```python
from build123d import *

# Parameters (mm, degrees)
SKETCH2_R = 65


with BuildPart() as part:
    # Sweep1: sweep along a path in Sketch1
    with BuildLine(Plane(origin=(0, 0, 0), x_dir=(0, 0, -1), z_dir=(1, 0, 0))) as sweep1_path:
        Line((-50, 0), (50, 0))
        Line((50, 0), (50, 120))
    # Sketch2 → Sweep1 (sweep)
    with BuildSketch(Plane.XY.offset(50)):
        Circle(SKETCH2_R)
    sweep1 = sweep(path=sweep1_path.line, transition=Transition.RIGHT)

    # Mirror1: Sweep1 across plane
    add(sweep1.mirror(Plane.XY.offset(-50)))


solid = part.part
```
Can you work these out from the model? Positions are in its coordinate system, mm. A direction names the side the tool comes from. Coordinates: 2 decimals unless noted, no trailing zeros. Loops run counter-clockwise (first coordinate to the right, second up) from the corner with the lowest first, then second, coordinate; pieces in that order, holes last. Notation, with made-up numbers: (81, 28) -> (105, 28) arc R21 cw to (105, 35) -> close; hole circle Ø3 at (-28, 41.5). An arc over 180 degrees is marked (long way). Answer as a JSON object with one key per item and string values.
1) Imagine slicing it at D-D (y = 68). Please give me the cut outline in (x, z).
Results:
{"outline": "circle Ø130 at (0, -50)"}
2) Imagine slicing it at B-B (x = 0). Please give me the cut outline in (y, z), then the cut area to 4 significant figures.
Results:
{"outline": "(-65, -150) -> (65, -150) -> (65, -115) -> (120, -115) -> (120, 15) -> (65, 15) -> (65, 50) -> (-65, 50) -> close", "area": "33,150 mm^2"}
3) Imagine slicing it at C-C (z = 6). Please give me the cut outline in (x, y).
Results:
{"outline": "(-33, 56) arc R65 ccw (long way) to (33, 56) -> (33, 120) -> (-33, 120) -> close"}
4) For faces 1 (the face through (1, 120, -49)), 2 (the face through (-47.91, 74.17, -93.93)), which set-ups out of +Z, -Z, +X, -X, +Y, -Y let a thin tool reach every point of the face, with its end or its side?
Results:
{"face 1": "+Z, -Z, +X, -X, +Y", "face 2": "+Y"}
5) If I drill on line 1 (X direction, y = 76.5, z = -50.5); line 2 (Y direction, x = 30, z = -64); line 3 (Y direction, x = -51.5, z = 3.5), over which ranges is the centre line in solid material (lowest first)?
Results:
{"line 1": "x = -65 to 65", "line 2": "y = -57.66 to 120", "line 3": "y = -39.66 to 39.66"}
6) Imagine slicing it at A-A (y = 44). Please give me the cut outline in (x, z).
Results:
{"outline": "(-47.84, -150) -> (47.84, -150) -> (47.84, -94) arc R65 ccw to (47.84, -6) -> (47.84, 50) -> (-47.84, 50) -> (-47.84, -6) arc R65 ccw to (-47.84, -94) -> close"}
7) For P1, Ø5, axis at x = 7.5, z = -5, coming from the -Y side; P2, Ø10, axis at x = 45.5, z = 2, coming from the -Y side; P3, Ø10, axis at y = -33, z = -120.5, coming from the -X side, each with a flat end and sliding along its axis, tell me the tip position at first contact or that it passes through.
Results:
{"P1": "stops at y = -64.81", "P2": "stops at y = -50.84", "P3": "stops at x = -58.66"}
